Build history of the part. All positions in model axes, mm. Face numbers are marked on the shaded views. Give positions to 0.01 mm unless a question says otherwise; leave off trailing zeros. Write each loop counter-clockwise with the first axis right and the second up, starting at its lowest first coordinate (ties: lowest second). Pieces come first, ordered by that corner, then holes. Notation, with made-up numbers: (-26, 29.5) -> (12, 29.5) arc R22 cw to (12, 66.5) -> close; hole circle Ø3 at (10, -39). An arc over 180 degrees is marked (long way). Put each result on its own line as item: value. Start each with the question number.
Item 1: Slice it at A-A, the plane z = -19. List the corners of the cut face in (x, y), plus the area to 3 significant figures.
Item 2: Two-plate mould, pull along Y, no slides. Class the marked faces 1, 2 and 3: pulls with the +Y half, pulls with the -Y half, needs draft (parallel to the pull), parting line crosses it, or undercut.
Item 3: Flat gauge pins, fed straight in: pin 1 Ø10 at (x, y) = (37.5, 44.5) entering from +Z; pin 2 Ø8 at (y, z) = (30.5, -30) entering from +X; pin 3 Ø4 at (x, y) = (-26, 63.5) entering from +Z; pin 4 Ø6 at (x, z) = (-21, -37.5) entering from -Y. Where does each tip first touch, or does it go through?
Item 4: Drill centre lines: line 1 along Y through (x, z) = (0, -38); line 2 along Y through (x, z) = (0, -24.5); line 3 along Z through (x, y) = (-43, -26.5). Where is each one in solid material? Low to high.
```python
from build123d import *

# Parameters (mm, degrees)
CHAMFER1_SIZE = 0.5
FILLET1_R     = 5
FILLET2_R     = 0.5


with BuildPart() as part:
    # Sketch1 → Revolve1 (revolve)
    with BuildSketch(Plane(origin=(0, 0, 0), x_dir=(1, 0, 0), z_dir=(0, 1, 0))):
        Polygon((69.75, 0), (76.25, 0), (76.25, 10), (73.75, 10), (73.75, 14.25), (76.25, 14.25), (76.25, 24.25), (73.75, 24.25), (73.75, 28.5), (76.25, 28.5), (76.25, 38.5), (73.75, 38.5), (73.75, 42.75), (76.25, 42.75), (76.25, 52.75), (82.55, 52.75), (82.55, 60.25), (0, 60.25), (0, 52.75), (69.75, 52.75), align=None)
    revolve(axis=Axis((0, 0, 0), (0, 0, -1)))

    # Chamfer1
    chamfer1_edges = [part.edges().sort_by_distance(p)[0] for p in [
        (-76.25, 0, -14.25),
        (-76.25, 0, -24.25),
        (-76.25, 0, -28.5),
        (-76.25, 0, -38.5),
        (-76.25, 0, -42.75),
        (-76.25, 0, -10),
    ]]
    chamfer(chamfer1_edges, length=CHAMFER1_SIZE)

    # Fillet1
    fillet1_edges = [part.edges().sort_by_distance(p)[0] for p in [
        (-76.25, 0, 0),
    ]]
    fillet(fillet1_edges, radius=FILLET1_R)

    # Fillet2
    fillet2_edges = [part.edges().sort_by_distance(p)[0] for p in [
        (-69.75, 0, 0),
    ]]
    fillet(fillet2_edges, radius=FILLET2_R)


solid = part.part
```
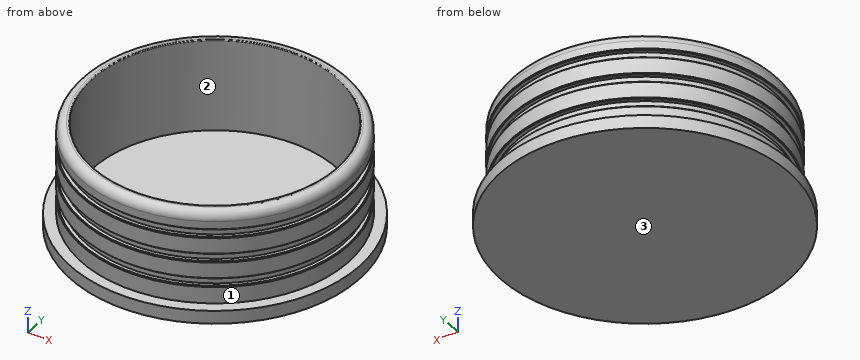
Values follow:
1. outline: circle Ø152.5 at (0, 0); hole circle Ø139.5 at (0, 0)
1. area: 2,980 mm2
2. face 1: parting line crosses it
2. face 2: undercut
2. face 3: needs draft
3. pin 1: z = -52.75
3. pin 2: x = 71.5
3. pin 3: z = 0
3. pin 4: y = -74.09
4. line 1: -76.25 to -69.75, 69.75 to 76.25
4. line 2: -73.75 to -69.75, 69.75 to 73.75
4. line 3: -60.25 to -52.75
